For this review, take the finished solid that the model builds, in its own axes (mm). Coordinates: 2 decimals unless noted, no trailing zeros. Loops run counter-clockwise (first coordinate to the right, second up) from the corner with the lowest first, then second, coordinate; pieces in that order, holes last. Notation, with made-up numbers: M -17,-2 L -7,-2 A28 ccw -7,23 Z; hole C 84.5,43 d1. An arc over 180 degrees is marked long. Put each result on its own line as item: value.
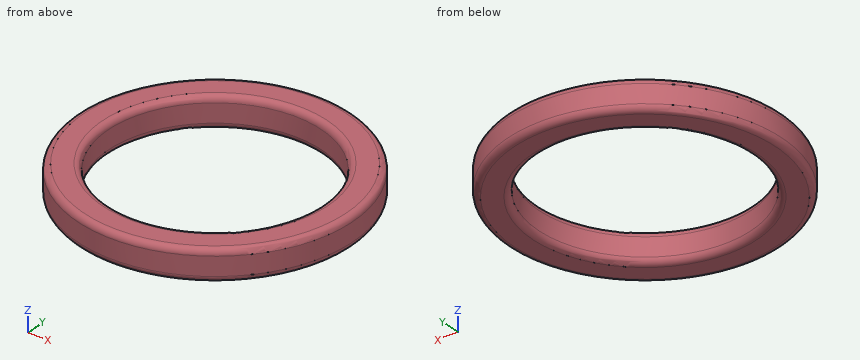
```python
from build123d import *

# Parameters (mm, degrees)
SKETCH1_R           = 22.612840435
SKETCH1_R_2         = 17.532840435
EXTRUDE_THIN1_DEPTH = 5.08
FILLET1_R           = 1


with BuildPart() as part:
    # Sketch1 → Extrude-Thin1 (new body)
    with BuildSketch(Plane.XY):
        with Locations((39.784875199, 9.634635023)):
            Circle(SKETCH1_R)
        with Locations((39.784875199, 9.634635023)):
            Circle(SKETCH1_R_2, mode=Mode.SUBTRACT)
    extrude(amount=EXTRUDE_THIN1_DEPTH)

    # Fillet1
    fillet1_edges = [part.edges().sort_by_distance(p)[0] for p in [
        (17.172034764, 9.634635023, 0),
        (17.172034764, 9.634635023, 5.08),
        (22.252034764, 9.634635023, 0),
        (22.252034764, 9.634635023, 5.08),
    ]]
    fillet(fillet1_edges, radius=FILLET1_R)


solid = part.part
```
(1) For pin 1 (21 mm diameter, centred on x = 39.78, y = 9.63, fed in from +Z); pin 2 (2 mm diameter, centred on x = 47.5, z = 4, fed in from -Y), all flat-tipped, find the tip position at first contact; note any pin that passes through.
Determined:
pin 1: passes through
pin 2: stops at y = -11.96
(2) Add section A-A (z = 1.85). Write out the cut boundary in (x, y).
Determined:
outline: C 39.78,9.63 d45.23; hole C 39.78,9.63 d35.07
(3) Wall thickness on line 1 along X through (y, z) = (9.5, 2.8); line 2 along X through (y, z) = (-4, 0.35); line 3 along Y through (x, z) = (53, 3.5): over which ranges is each line inside the solid? List them lowest first. Write a range as [from, to].
Determined:
line 1: x = [17.17, 22.25], [57.32, 62.4]
line 2: x = [22.05, 28.38], [51.19, 57.52]
line 3: y = [-8.71, -1.89], [21.16, 27.98]
